from build123d import *

# Parameters (mm, degrees)
IZIM1_R                     = 148
Y_KSEKLIK_EKSTR_ZYON1_DEPTH = 60
Y_KSEKLIK_EKSTR_ZYON2_START = 10
IZIM2_R                     = 167.5
Y_KSEKLIK_EKSTR_ZYON2_DEPTH = 50
IZIM3_R                     = 55
KES_EKSTR_ZYON1_DEPTH       = 741
Y_KSEKLIK_EKSTR_ZYON3_START = -50
IZIM4_R                     = 55
IZIM4_R_2                   = 38.5
Y_KSEKLIK_EKSTR_ZYON3_DEPTH = 10
IZIM5_R                     = 167.5
IZIM5_R_2                   = 38.5
Y_KSEKLIK_EKSTR_ZYON4_DEPTH = 5
IZIM6_R                     = 60.5
IZIM6_R_2                   = 54.5
KES_EKSTR_ZYON2_DEPTH       = 10
IZIM7_R                     = 4
KES_EKSTR_ZYON3_DEPTH       = 55
IZIM8_R                     = 7
KES_EKSTR_ZYON4_DEPTH       = 17
RADYUS1_R                   = 15
RADYUS2_R                   = 2


with BuildPart() as part:
    # Çizim1 → Yükseklik-Ekstrüzyon1 (new body)
    with BuildSketch(Plane.XY):
        Circle(IZIM1_R)
    extrude(amount=Y_KSEKLIK_EKSTR_ZYON1_DEPTH)

    # Çizim2 → Yükseklik-Ekstrüzyon2 (add)
    with BuildSketch(Plane.XY.offset(Y_KSEKLIK_EKSTR_ZYON2_START)):
        Circle(IZIM2_R)
    extrude(amount=Y_KSEKLIK_EKSTR_ZYON2_DEPTH)

    # Çizim3 → Kes-Ekstrüzyon1 (cut)
    with BuildSketch(Plane(origin=(0, 0, 0), x_dir=(-1, 0, 0), z_dir=(0, 0, -1))):
        Circle(IZIM3_R)
    extrude(amount=-KES_EKSTR_ZYON1_DEPTH, mode=Mode.SUBTRACT)

    # Çizim4 → Yükseklik-Ekstrüzyon3 (add)
    with BuildSketch(Plane(origin=(0, 0, 0), x_dir=(-1, 0, 0), z_dir=(0, 0, -1)).offset(Y_KSEKLIK_EKSTR_ZYON3_START)):
        Circle(IZIM4_R)
        Circle(IZIM4_R_2, mode=Mode.SUBTRACT)
    extrude(amount=-Y_KSEKLIK_EKSTR_ZYON3_DEPTH)

    # Çizim5 → Yükseklik-Ekstrüzyon4 (add)
    with BuildSketch(Plane.XY.offset(60)):
        Circle(IZIM5_R)
        with Locations(Location((0, 0, 0), (0, 0, 180))):
            Circle(IZIM5_R_2, mode=Mode.SUBTRACT)
    extrude(amount=Y_KSEKLIK_EKSTR_ZYON4_DEPTH)

    # Çizim6 → Kes-Ekstrüzyon2 (cut)
    with BuildSketch(Plane.XY.offset(65)):
        Circle(IZIM6_R)
        Circle(IZIM6_R_2, mode=Mode.SUBTRACT)
    extrude(amount=-KES_EKSTR_ZYON2_DEPTH, mode=Mode.SUBTRACT)

    # Çizim7 → Kes-Ekstrüzyon3 (cut)
    with BuildSketch(Plane.XY.offset(65)):
        with Locations((-107.349895203, 112.5)):
            Circle(IZIM7_R)
        with Locations((107.349895203, 112.5)):
            Circle(IZIM7_R)
        with Locations((107.349895203, -112.5)):
            Circle(IZIM7_R)
        with Locations((-107.349895203, -112.5)):
            Circle(IZIM7_R)
    extrude(amount=-KES_EKSTR_ZYON3_DEPTH, mode=Mode.SUBTRACT)

    # Çizim8 → Kes-Ekstrüzyon4 (cut)
    with BuildSketch(Plane.XY.offset(65)):
        with Locations((-107.349895203, 112.5)):
            Circle(IZIM8_R)
        with Locations((107.349895203, 112.5)):
            Circle(IZIM8_R)
        with Locations((107.349895203, -112.5)):
            Circle(IZIM8_R)
        with Locations((-107.349895203, -112.5)):
            Circle(IZIM8_R)
    extrude(amount=-KES_EKSTR_ZYON4_DEPTH, mode=Mode.SUBTRACT)

    # Radyus1
    # the kernel refuses this fillet: 15 mm, written as the material it takes off along each edge
    with BuildSketch(Plane(origin=(0, 0, 65), x_dir=(1, 0, 0), z_dir=(0, -1, 0))) as radyus1_piece_1:
        with BuildLine():
            CenterArc((167.5 - RADYUS1_R, -RADYUS1_R), RADYUS1_R, 0, 90)
            Line((167.5 - RADYUS1_R, 0), (167.5, 0))
            Line((167.5, 0), (167.5, -RADYUS1_R))
        make_face()
    revolve(axis=Axis((0, 0, 65), (0, 0, 1)), mode=Mode.SUBTRACT)

    # Radyus2
    radyus2_edges = [part.edges().sort_by_distance(p)[0] for p in [
        (38.5, 0, 65),
        (-60.5, 0, 65),
        (-54.5, 0, 65),
    ]]
    fillet(radyus2_edges, radius=RADYUS2_R)


solid = part.part
CAD build for the part. Positions are in the model's coordinates, mm. A direction names the side the tool comes from. Give positions to 0.01 mm unless a question says otherwise; leave off trailing zeros. Order: outer loops, then holes, each group sorted by start corner. A loop starts at its lowest first (then second) coordinate and runs counter-clockwise, first axis right, second up. Notation, with made-up numbers: (80.5, 35.5) -> (128.5, 35.5) arc R21 ccw to (128.5, 53.5) -> close; hole circle Ø11 at (59.5, 58). An arc over 180 degrees is marked (long way). Return JSON: item names as keys, results as strings.
Q1. Drill centre lines: line 1 (X direction, y = 6.5, z = 61); line 2 (Y direction, x = -109, z = 34); line 3 (X direction, y = 112, z = 29). Where is each one in solid material? Low to high.
Working result:
{"line 1": "-162.57 to -60.15, -54.11 to -37.95, 37.95 to 54.11, 60.15 to 162.57", "line 2": "-127.18 to -116.14, -108.86 to 108.86, 116.14 to 127.18", "line 3": "-124.55 to -111.32, -103.38 to 103.38, 111.32 to 124.55"}
Q2. Mould opens along X. For faces 1 (the face through (66, 2, 65)), 2 (the face through (110, 109, 48)), 3 (the face through (-32.08, -144.48, 4.93)) say: pulls with the +X half, pulls with the -X half, needs draft (parallel to the pull), parting line crosses it, or undercut.
Working result:
{"face 1": "needs draft", "face 2": "undercut", "face 3": "parting line crosses it"}
Q3. Which spindle directions (+Z, -Z, +X, -X, +Y, -Y) get a long thin tool onto all of the face, cutting with end or side? Do faces 4 (the face through (-103.535, -111.299, 29.266)), 5 (the face through (11.923, -53.692, 24.65)), 6 (the face through (-103.587, -106.598, 56.619)). Say none if no direction does.
Working result:
{"face 4": "+Z, -Z", "face 5": "-Z", "face 6": "+Z"}
Q4. Saw through at C-C (z = 27). Write the cut outline in (x, y), then the cut area to 3 significant figures.
Working result:
{"outline": "circle Ø335 at (0, 0); hole circle Ø8 at (-107.35, -112.5); hole circle Ø8 at (-107.35, 112.5); hole circle Ø110 at (0, 0); hole circle Ø8 at (107.35, -112.5); hole circle Ø8 at (107.35, 112.5)", "area": "78,400 mm²"}
Q5. Flat gauge pins, fed straight in: pin 1 (4 mm diameter, centred on x = 108, y = 116, fed in from +Z); pin 2 (2 mm diameter, centred on x = 67.5, z = 41.5, fed in from +Y); pin 3 (5 mm diameter, centred on x = 61.5, z = 54, fed in from +Y); pin 4 (18 mm diameter, centred on x = -107.35, y = -112.5, fed in from -Z). Where does each tip first touch, or does it go through?
Working result:
{"pin 1": "z = 48", "pin 2": "y = 153.73", "pin 3": "y = 156.37", "pin 4": "z = 0"}
